Can you work these out from the model? Positions are in its coordinate system, mm. A direction names the side the tool comes from. Round coordinates to 2 decimals unless told otherwise and drop trailing zeros. Loops run counter-clockwise (first coordinate to the right, second up) from the corner with the lowest first, then second, coordinate; pieces in that order, holes last. Notation, with made-up numbers: M 62.25,-5 L 87.25,-5 A21 cw 87.25,4 Z; hole C 21,48.25 d2. An arc over 180 degrees is marked long. Return JSON: item names as keys, results as strings.
```python
from build123d import *

# Parameters (mm, degrees)
F0_W     = 32
F0_H     = 16
F1_DEPTH = 10
F2_T     = -1.5
F3_R     = 2.425
F4_DEPTH = 1.6
F5_R     = 2.925
F6_DEPTH = 10


with BuildPart() as f1:
    # F0 (on Top) → F1 (new body)
    with BuildSketch(Plane.XY):
        Rectangle(F0_W, F0_H)
    extrude(amount=F1_DEPTH)

    # F2
    f2_openings = [f1.faces().sort_by_distance(p)[0] for p in [
        (0, 0, 0),
    ]]
    offset(amount=F2_T, openings=f2_openings)

    # F3 (on face) → F4 (join)
    with BuildSketch(Plane.XY.offset(10)):
        with Locations((-12, -4)):
            Circle(F3_R)
        with Locations((-12, 4)):
            Circle(F3_R)
        with Locations((-4, -4)):
            Circle(F3_R)
        with Locations((-4, 4)):
            Circle(F3_R)
        with Locations((4, -4)):
            Circle(F3_R)
        with Locations((4, 4)):
            Circle(F3_R)
        with Locations((12, -4)):
            Circle(F3_R)
        with Locations((12, 4)):
            Circle(F3_R)
    extrude(amount=F4_DEPTH)

    # F5 (on face) → F6 (join)
    with BuildSketch(Plane.XY.offset(10)):
        with Locations((-10.257971, 0)):
            Circle(F5_R)
        with BuildLine():
            ThreePointArc((12.301918, 0), (9.376918, 2.925), (6.451918, 0))
            ThreePointArc((6.451918, 0), (9.376918, -2.925), (12.301918, 0))
        make_face()
        with BuildLine():
            ThreePointArc((2.925, 0), (0, 2.925), (-2.925, 0))
            Line((-2.925, 0), (0, 0))
            Line((0, 0), (2.925, 0))
        make_face()
        with BuildLine():
            Line((0, 0), (-2.925, 0))
            ThreePointArc((-2.925, 0), (0, -2.925), (2.925, 0))
            Line((2.925, 0), (0, 0))
        make_face()
    extrude(amount=F6_DEPTH)


solid = f1.part
```
Q1. Suppose I cut it at A-A, the plane x = 0. Please give me the cut outline in (y, z) (3 decimals), plus the area to 3 significant figures.
Results:
{"outline": "M -8,0 L -6.5,0 L -6.5,8.5 L 6.5,8.5 L 6.5,0 L 8,0 L 8,10 L 2.925,10 L 2.925,20 L -2.925,20 L -2.925,10 L -8,10 Z", "area": "108 mm2"}
Q2. Suppose I cut it at C-C, the plane z = 3.5. Please give me the cut outline in (x, y), plus the area to 3 significant figures.
Results:
{"outline": "M -16,-8 L 16,-8 L 16,8 L -16,8 Z; hole M -14.5,-6.5 L 14.5,-6.5 L 14.5,6.5 L -14.5,6.5 Z", "area": "135 mm2"}
Q3. Thinking about a two-plate mould opening in Y: for faces 1 (the flat face through (0, -8, 5)), 2 (the flat face through (0, -6.5, 4)), 3 (the flat face through (12, -4, 11.6)), 4 (the flat face through (0, 8, 5)), which applies, pulls with the +Y half, pulls with the -Y half, needs draft (parallel to the pull), parting line crosses it, or undercut?
Results:
{"face 1": "pulls with the -Y half", "face 2": "undercut", "face 3": "needs draft", "face 4": "pulls with the +Y half"}
Q4. Suppose I cut it at B-B, the plane z = 11.25. Please give me the cut outline in (x, y) (3 decimals), plus the area to 3 significant figures.
Results:
{"outline": "M -12.661,-1.667 A2.425 ccw long -9.841,-2.895 A2.925 ccw -9.841,2.895 A2.425 ccw long -12.661,1.667 A2.925 ccw Z; C -4,-4 d4.85; C -4,4 d4.85; C 0,0 d5.85; C 4,-4 d4.85; C 4,4 d4.85; M 9.845,-2.887 A2.425 ccw long 11.838,-1.58 A2.925 ccw 11.838,1.58 A2.425 ccw long 9.845,2.887 A2.925 ccw long Z", "area": "222 mm2"}
Q5. On a 3-axis mill with a long thin cutter (end or side, diameter ignored), from which of +Z, -Z, +X, -X, +Y, -Y can I reach the whole of each face in a straight line? I mean faces 5 (the flat face through (-14.5, 0, 4)), 6 (the flat face through (-4, 4, 11.6)), 7 (the cylindrical face through (6.313, -3.272, 10.789)). Say none if no direction works.
Results:
{"face 5": "-Z", "face 6": "+Z, +Y", "face 7": "+Z"}
Q6. If I drill on line 1 along Y through (x, z) = (-12, 4.25); line 2 along X through (y, z) = (0.25, 14.75); line 3 along X through (y, z) = (1.75, 3), over which ranges is the centre line in solid material (lowest first)?
Results:
{"line 1": "y = -8 to -6.5, 6.5 to 8", "line 2": "x = -13.17 to -7.34, -2.91 to 2.91, 6.46 to 12.29", "line 3": "x = -16 to -14.5, 14.5 to 16"}
Q7. I'm going to push flat-ended pins straight in: pin 1 Ø1.4 at (x, y) = (-12, -4) entering from +Z; pin 2 Ø2.5 at (x, y) = (11, 3.5) entering from +Z; pin 3 Ø2 at (x, y) = (5, -2) entering from -Z; pin 4 Ø1 at (x, z) = (11.5, 15) entering from +Y. Where does each tip first touch, or does it pass through?
Results:
{"pin 1": "stops at z = 11.6", "pin 2": "stops at z = 20", "pin 3": "stops at z = 8.5", "pin 4": "stops at y = 2.43"}
Q8. Suppose I cut it at D-D, the plane y = 4. Please give me the cut outline in (x, z) (3 decimals).
Results:
{"outline": "M -16,0 L -14.5,0 L -14.5,8.5 L 14.5,8.5 L 14.5,0 L 16,0 L 16,10 L 14.425,10 L 14.425,11.6 L 9.575,11.6 L 9.575,10 L 6.425,10 L 6.425,11.6 L 1.575,11.6 L 1.575,10 L -1.575,10 L -1.575,11.6 L -6.425,11.6 L -6.425,10 L -9.575,10 L -9.575,11.6 L -14.425,11.6 L -14.425,10 L -16,10 Z"}
